Check sheet for the modelled part. Datum: model origin and axes. Units: mm. A direction names the side the tool comes from. Give positions to 0.01 mm unless a question says otherwise; leave off trailing zeros. Loops run counter-clockwise (first coordinate to the right, second up) from the corner with the lowest first, then second, coordinate; pieces in that order, holes last. Notation, with made-up numbers: (72.25, 47) - (130.25, 47) arc R36 cw to (130.25, 82) - close; hole circle Ø11 at (15.25, 6.5). An arc over 180 degrees is marked (long way). Answer in a Markdown table with one row per item. Add a question column.
(1) Set-up check for faces 4 (the face through (-39, 35, 2.381)), 5 (the face through (-1, 0, 2.381)), 6 (the face through (-1, 1, 0)): record each of +Z, -Z, +X, -X, +Y, -Y from which the full face is reachable in a straight line by a thin tool's end or side.
(2) Sectioned sample at A-A on x = 29.5. Enter the section's corners in (y, z) (1 decimal).
(3) Thickness scan on L1, parallel to X at y = -26.5, z = 4.5 (3 decimals); L2, parallel to Y at x = -9, z = 4.3 (3 decimals); L3, parallel to X at y = -35, z = 1.6 (3 decimals). Record the ranges inside material, lowest first.
(4) Go/stop test with a flat-tipped pin: P1, Ø5, axis at x = 41.275, y = -34.925, coming from the -Z side. Record where the tip stops, or that it passes through.
(5) Sectioned sample at B-B on y = -9. Enter the section's corners in (x, z) (1 decimal).
(6) Draft check along X on faces 1 (the face through (-39.69, 34.27, 3.56)), 2 (the face through (-47.625, -1, 3)), 3 (the face through (-1, -41.275, 3)). Enter one of: released by +X, released by -X, zero draft, split by the parting line, or undercut.
from build123d import *

# Parameters (mm, degrees)
SKETCH1_W                                  = 95.25
SKETCH1_H                                  = 82.55
BOSS_EXTRUDE1_DEPTH                        = 4.7625
SKETCH2_W                                  = 92.338000236
SKETCH2_H                                  = 79.638
SKETCH2_W_2                                = 88.392
SKETCH2_H_2                                = 75.692
CUT_EXTRUDE1_DEPTH                         = 1.8415
FILLET1_R                                  = 1.5875
FILLET2_R                                  = 1.5875
SKETCH3_R                                  = 1.7145
CUT_EXTRUDE2_DEPTH                         = 64.201642829
SKETCH4_R                                  = 3.048
CUT_EXTRUDE3_DEPTH                         = 2.38125
MIRROR1_AT_THE_SECOND_PLANE_COPY_1_SKETC_R = 1.7145
MIRROR1_AT_THE_SECOND_PLANE_COPY_1_DEPTH   = 64.201642829
MIRROR1_AT_THE_SECOND_PLANE_COPY_2_SKETC_R = 3.048
MIRROR1_AT_THE_SECOND_PLANE_COPY_2_DEPTH   = 2.38125
CUT_EXTRUDE4_DEPTH                         = 2.38125


with BuildPart() as part:
    # Sketch1 → Boss-Extrude1 (new body)
    with BuildSketch(Plane.XY):
        Rectangle(SKETCH1_W, SKETCH1_H)
    extrude(amount=BOSS_EXTRUDE1_DEPTH)

    # Sketch2 → Cut-Extrude1 (cut)
    with BuildSketch(Plane.XY.offset(4.7625)):
        Rectangle(SKETCH2_W, SKETCH2_H)
        Rectangle(SKETCH2_W_2, SKETCH2_H_2, mode=Mode.SUBTRACT)
    extrude(amount=-CUT_EXTRUDE1_DEPTH, mode=Mode.SUBTRACT)

    # Fillet1
    fillet1_edges = [part.edges().sort_by_distance(p)[0] for p in [
        (46.169000118, 39.819, 3.84175),
        (46.169000118, -39.819, 3.84175),
        (-46.169000118, -39.819, 3.84175),
        (-46.169000118, 39.819, 3.84175),
        (44.196, -37.846, 3.84175),
        (-44.196, -37.846, 3.84175),
        (-44.196, 37.846, 3.84175),
        (44.196, 37.846, 3.84175),
    ]]
    fillet(fillet1_edges, radius=FILLET1_R)

    # Fillet2
    fillet2_edges = [part.edges().sort_by_distance(p)[0] for p in [
        (0, -41.275, 0),
        (-47.625, 0, 0),
        (0, 41.275, 0),
        (47.625, 0, 0),
        (47.625, -41.275, 2.38125),
        (-47.625, -41.275, 2.38125),
        (-47.625, 41.275, 2.38125),
        (47.625, 41.275, 2.38125),
    ]]
    fillet(fillet2_edges, radius=FILLET2_R)

    # Sketch3 → Cut-Extrude2 (cut, through all)
    with BuildSketch(Plane(origin=(0, 0, 0), x_dir=(-1, 0, 0), z_dir=(0, 0, -1))):
        with Locations((-41.275, 34.925)):
            Circle(SKETCH3_R)
    cut_extrude2 = extrude(amount=-CUT_EXTRUDE2_DEPTH, mode=Mode.SUBTRACT)

    # Sketch4 → Cut-Extrude3 (cut)
    with BuildSketch(Plane(origin=(0, 0, 0), x_dir=(-1, 0, 0), z_dir=(0, 0, -1))):
        with Locations((-41.275, 34.925)):
            Circle(SKETCH4_R)
    cut_extrude3 = extrude(amount=-CUT_EXTRUDE3_DEPTH, mode=Mode.SUBTRACT)

    # Mirror1: Cut-Extrude2, Cut-Extrude3 across plane
    add(cut_extrude2.mirror(Plane(origin=(0, 0, 0), x_dir=(0, 0, 1), z_dir=(1, 0, 0))), mode=Mode.SUBTRACT)
    add(cut_extrude3.mirror(Plane(origin=(0, 0, 0), x_dir=(0, 0, 1), z_dir=(1, 0, 0))), mode=Mode.SUBTRACT)

    # Mirror1 at the second plane: Cut-Extrude2, Cut-Extrude3 across plane
    add(cut_extrude2.mirror(Plane.ZX), mode=Mode.SUBTRACT)
    add(cut_extrude3.mirror(Plane.ZX), mode=Mode.SUBTRACT)

    # Mirror1 at the second plane copy 1 sketc → Mirror1 at the second plane copy 1 (cut, through all)
    with BuildSketch(Plane(origin=(0, 0, 0), x_dir=(1, 0, 0), z_dir=(0, 0, -1))):
        with Locations((-41.275, 34.925)):
            Circle(MIRROR1_AT_THE_SECOND_PLANE_COPY_1_SKETC_R)
    extrude(amount=-MIRROR1_AT_THE_SECOND_PLANE_COPY_1_DEPTH, mode=Mode.SUBTRACT)

    # Mirror1 at the second plane copy 2 sketc → Mirror1 at the second plane copy 2 (cut)
    with BuildSketch(Plane(origin=(0, 0, 0), x_dir=(1, 0, 0), z_dir=(0, 0, -1))):
        with Locations((-41.275, 34.925)):
            Circle(MIRROR1_AT_THE_SECOND_PLANE_COPY_2_SKETC_R)
    extrude(amount=-MIRROR1_AT_THE_SECOND_PLANE_COPY_2_DEPTH, mode=Mode.SUBTRACT)

    # Sketch5 → Cut-Extrude4 (cut)
    with BuildSketch(Plane.XY.offset(4.7625)):
        with BuildLine():
            Line((-36.2585, -31.496), (36.2585, -31.496))
            ThreePointArc((36.2585, -31.496), (37.381032015, -31.031032015), (37.846, -29.9085))
            Line((37.846, -29.9085), (37.846, 29.9085))
            ThreePointArc((37.846, 29.9085), (37.381032015, 31.031032015), (36.2585, 31.496))
            Line((36.2585, 31.496), (-36.2585, 31.496))
            ThreePointArc((-36.2585, 31.496), (-37.381032015, 31.031032015), (-37.846, 29.9085))
            Line((-37.846, 29.9085), (-37.846, -29.9085))
            ThreePointArc((-37.846, -29.9085), (-37.381032015, -31.031032015), (-36.2585, -31.496))
        make_face()
    extrude(amount=-CUT_EXTRUDE4_DEPTH, mode=Mode.SUBTRACT)


solid = part.part
Reply:
| question | item | result |
|---|---|---|
| 1 | face 4 | -Z |
| 1 | face 5 | +Z |
| 1 | face 6 | -Z, +X, -X, +Y, -Y |
| 2 | outline | (-41.3, 1.6) arc R1.6 ccw to (-39.7, 0) - (39.7, 0) arc R1.6 ccw to (41.3, 1.6) - (41.3, 4.8) - (39.8, 4.8) - (39.8, 2.9) - (37.8, 2.9) - (37.8, 4.8) - (31.5, 4.8) - (31.5, 2.4) - (-31.5, 2.4) - (-31.5, 4.8) - (-37.8, 4.8) - (-37.8, 2.9) - (-39.8, 2.9) - (-39.8, 4.8) - (-41.3, 4.8) - close |
| 3 | L1 | -47.625 to -46.169, -44.196 to -37.846, 37.846 to 44.196, 46.169 to 47.625 |
| 3 | L2 | -41.275 to -39.819, -37.846 to -31.496, 31.496 to 37.846, 39.819 to 41.275 |
| 3 | L3 | -47.625 to -44.322, -38.228 to 38.228, 44.322 to 47.625 |
| 4 | P1 | z = 2.38 |
| 5 | outline | (-47.6, 1.6) arc R1.6 ccw to (-46, 0) - (46, 0) arc R1.6 ccw to (47.6, 1.6) - (47.6, 4.8) - (46.2, 4.8) - (46.2, 2.9) - (44.2, 2.9) - (44.2, 4.8) - (37.8, 4.8) - (37.8, 2.4) - (-37.8, 2.4) - (-37.8, 4.8) - (-44.2, 4.8) - (-44.2, 2.9) - (-46.2, 2.9) - (-46.2, 4.8) - (-47.6, 4.8) - close |
| 6 | face 1 | undercut |
| 6 | face 2 | released by -X |
| 6 | face 3 | zero draft |
